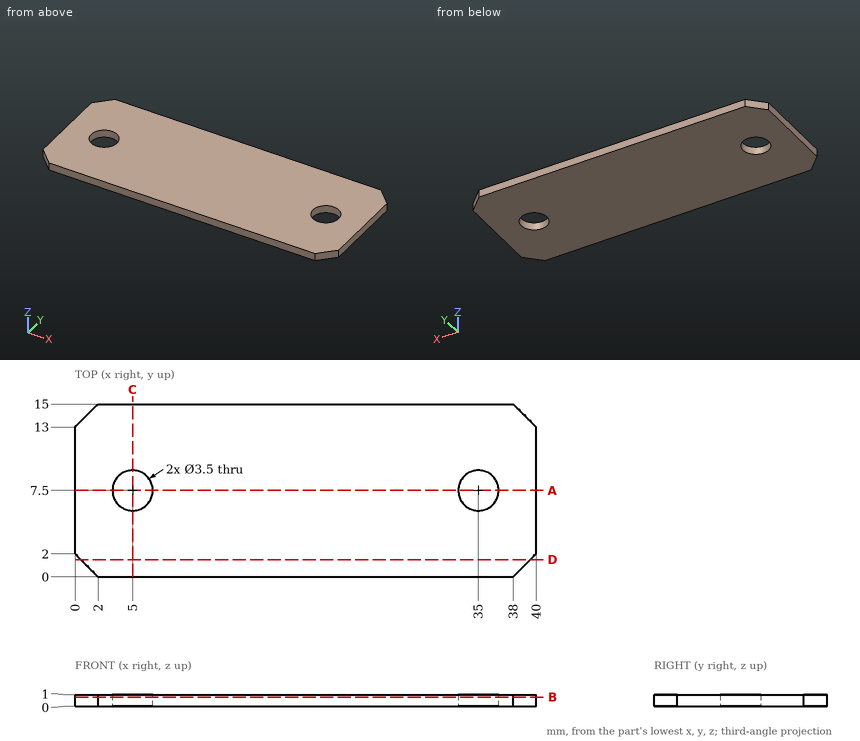
Input: dimensioned drawing with shaded views. Units: mm. Origin: part minimum x, y, z. Coordinates: 2 decimals unless noted, no trailing zeros. Order: outer loops, then holes, each group sorted by start corner. A loop starts at its lowest first (then second) coordinate and runs counter-clockwise, first axis right, second up. Notation, with made-up numbers: (-30, 68.25) -> (0, 68.25) arc R36 ccw to (0, 103.25) -> close; hole circle Ø2 at (84.5, 66). An arc over 180 degrees is marked (long way). Answer in a Markdown table with one row per item.
Item 1: Section D-D on y = 1.5. Output: boundary loops of the cut face in (x, z), plus the area to 3 significant figures.
Return value:
| item | result |
|---|---|
| outline | (0.5, 0) -> (39.5, 0) -> (39.5, 1) -> (0.5, 1) -> close |
| area | 39.0 mm² |
Item 2: Section B-B on z = 0.8. Output: boundary loops of the cut face in (x, y).
Return value:
| item | result |
|---|---|
| outline | (0, 2) -> (2, 0) -> (38, 0) -> (40, 2) -> (40, 13) -> (38, 15) -> (2, 15) -> (0, 13) -> close; hole circle Ø3.5 at (5, 7.5); hole circle Ø3.5 at (35, 7.5) |
Item 3: Section C-C on x = 5. Output: boundary loops of the cut face in (y, z), plus the area to 3 significant figures.
Return value:
| item | result |
|---|---|
| outline | (0, 0) -> (5.75, 0) -> (5.75, 1) -> (0, 1) -> close; (9.25, 0) -> (15, 0) -> (15, 1) -> (9.25, 1) -> close |
| area | 11.5 mm² |
Item 4: Section A-A on y = 7.5. Output: boundary loops of the cut face in (x, z), plus the area to 3 significant figures.
Return value:
| item | result |
|---|---|
| outline | (0, 0) -> (3.25, 0) -> (3.25, 1) -> (0, 1) -> close; (6.75, 0) -> (33.25, 0) -> (33.25, 1) -> (6.75, 1) -> close; (36.75, 0) -> (40, 0) -> (40, 1) -> (36.75, 1) -> close |
| area | 33.0 mm² |
Item 5: Ray query, L1, parallel to Y at x = 35, z = 0.65; L2, parallel to X at y = 7.75, z = 0.45; L3, parallel to Y at x = 6.5, z = 0.85. Return the intervals inside material, ascending.
Return value:
| item | result |
|---|---|
| L1 | y = 0 to 5.75, 9.25 to 15 |
| L2 | x = 0 to 3.27, 6.73 to 33.27, 36.73 to 40 |
| L3 | y = 0 to 6.6, 8.4 to 15 |
